CAD build for the part. Positions are in the model's coordinates, mm. Face numbers are marked on the shaded views. A direction names the side the tool comes from. Round coordinates to 2 decimals unless told otherwise and drop trailing zeros. Write each loop counter-clockwise with the first axis right and the second up, starting at its lowest first coordinate (ties: lowest second). Pieces come first, ordered by that corner, then holes. Notation, with made-up numbers: (51, 49) - (67, 49) arc R24 ccw to (67, 66) - close; hole circle Ø8 at (9, -36). An arc over 180 degrees is marked (long way). Use one line per item in the form item = value. Start each with the question number.
Item 1: Pull direction Z, two halves, no side cores. Call the marked faces 1, 2, 3 and 4: +Z half, -Z half, draft (parallel to the pull), parting line (faces both ways), or undercut.
Item 2: Band-saw the part on A-A, the plane x = -36. List the corners of the cut face in (y, z).
Item 3: Band-saw the part on D-D, the plane x = 1. List the corners of the cut face in (y, z).
Item 4: Band-saw the part on C-C, the plane z = -4.5. List the corners of the cut face in (x, y), and give its area (3 significant figures).
Item 5: Tool access for the marked faces 5, 6 and 7: list every direction of +Z, -Z, +X, -X, +Y, -Y with a clear straight run to the whole face (end or side of a thin tool).
Item 6: Drill centre lines: L1, parallel to X at y = 13, z = 30; L2, parallel to Z at x = -37, y = 12. Where is each one in solid material? Low to high.
Item 7: Pin check, flat tips, straight feed: pin 1 (4.5 mm diameter, centred on x = 37.5, z = -26.5, fed in from +Y); pin 2 (1.5 mm diameter, centred on y = 51, z = 21.5, fed in from +X); pin 3 (12 mm diameter, centred on x = -36.5, z = -33, fed in from +Y); pin 4 (3 mm diameter, centred on x = 27.5, z = -9.5, fed in from +Y). Stop position of each tip, or through.
Item 8: Band-saw the part on B-B, the plane y = 70. List the corners of the cut face in (x, z).
from build123d import *

# Parameters (mm, degrees)
BOSS_EXTRUDE1_DEPTH = 15
SKETCH1_5_R         = 7.5
CUT_EXTRUDE2_DEPTH  = 15
SKETCH1_6_R         = 7.5
SKETCH1_6_R_2       = 5.5
BOSS_EXTRUDE2_DEPTH = 10
BOSS_EXTRUDE3_DEPTH = 20


with BuildPart() as part:
    # Sketch1 → Boss-Extrude1 (new body)
    with BuildSketch(Plane(origin=(0, 0, 0), x_dir=(1, 0, 0), z_dir=(0, 1, 0))):
        with BuildLine():
            Line((52.75, -30), (52.75, 30))
            ThreePointArc((52.75, 30), (50.288021644, 38.233954897), (43.710264901, 43.765000629))
            Line((43.710264901, 43.765000629), (11.920529801, 57.530001258))
            ThreePointArc((11.920529801, 57.530001258), (0, 60), (-11.920529801, 57.530001258))
            Line((-11.920529801, 57.530001258), (-43.710264901, 43.765000629))
            ThreePointArc((-43.710264901, 43.765000629), (-50.288021644, 38.233954897), (-52.75, 30))
            Line((-52.75, 30), (-52.75, -30))
            ThreePointArc((-52.75, -30), (-48.356601718, -40.606601718), (-37.75, -45))
            Line((-37.75, -45), (37.75, -45))
            ThreePointArc((37.75, -45), (48.356601718, -40.606601718), (52.75, -30))
        make_face()
    extrude(amount=BOSS_EXTRUDE1_DEPTH)

    # Sketch1_5 → Cut-Extrude2 (cut)
    with BuildSketch(Plane(origin=(0, 0, 0), x_dir=(1, 0, 0), z_dir=(0, 1, 0))):
        with Locations((-37.75, 30)):
            Circle(SKETCH1_5_R)
        with Locations((37.75, 30)):
            Circle(SKETCH1_5_R)
        with Locations((37.75, -30)):
            Circle(SKETCH1_5_R)
        with Locations((-37.75, -30)):
            Circle(SKETCH1_5_R)
    extrude(amount=CUT_EXTRUDE2_DEPTH, mode=Mode.SUBTRACT)

    # Sketch1_6 → Boss-Extrude2 (add)
    with BuildSketch(Plane(origin=(0, 0, 0), x_dir=(1, 0, 0), z_dir=(0, 1, 0))):
        with Locations((-37.75, 30)):
            Circle(SKETCH1_6_R)
        with Locations((-37.75, 30)):
            Circle(SKETCH1_6_R_2, mode=Mode.SUBTRACT)
        with Locations((37.75, 30)):
            Circle(SKETCH1_6_R)
        with Locations((37.75, 30)):
            Circle(SKETCH1_6_R_2, mode=Mode.SUBTRACT)
        with Locations((37.75, -30)):
            Circle(SKETCH1_6_R)
        with Locations((37.75, -30)):
            Circle(SKETCH1_6_R_2, mode=Mode.SUBTRACT)
        with Locations((-37.75, -30)):
            Circle(SKETCH1_6_R)
        with Locations((-37.75, -30)):
            Circle(SKETCH1_6_R_2, mode=Mode.SUBTRACT)
    extrude(amount=BOSS_EXTRUDE2_DEPTH)

    # Sketch2 → Boss-Extrude3 (add, symmetric)
    with BuildSketch(Plane.XY):
        with BuildLine():
            Line((-25, 79), (-25, 76))
            ThreePointArc((-25, 76), (-25.292893219, 75.292893219), (-26, 75))
            Line((-26, 75), (-29.580398915, 75))
            ThreePointArc((-29.580398915, 75), (-26.457352845, 65.85756455), (-20.590457551, 58.181818182))
            ThreePointArc((-20.590457551, 58.181818182), (-14.516162744, 30.768138177), (-37.749172176, 15))
            Line((-37.749172176, 15), (37.749172176, 15))
            ThreePointArc((37.749172176, 15), (14.516162744, 30.768138177), (20.590457551, 58.181818182))
            ThreePointArc((20.590457551, 58.181818182), (26.457352845, 65.85756455), (29.580398915, 75))
            Line((29.580398915, 75), (26, 75))
            ThreePointArc((26, 75), (25.292893219, 75.292893219), (25, 76))
            Line((25, 76), (25, 79))
            ThreePointArc((25, 79), (24.707106781, 79.707106781), (24, 80))
            Line((24, 80), (22, 80))
            ThreePointArc((22, 80), (0, 58), (-22, 80))
            Line((-22, 80), (-24, 80))
            ThreePointArc((-24, 80), (-24.707106781, 79.707106781), (-25, 79))
        make_face()
    extrude(amount=BOSS_EXTRUDE3_DEPTH, both=True)


solid = part.part
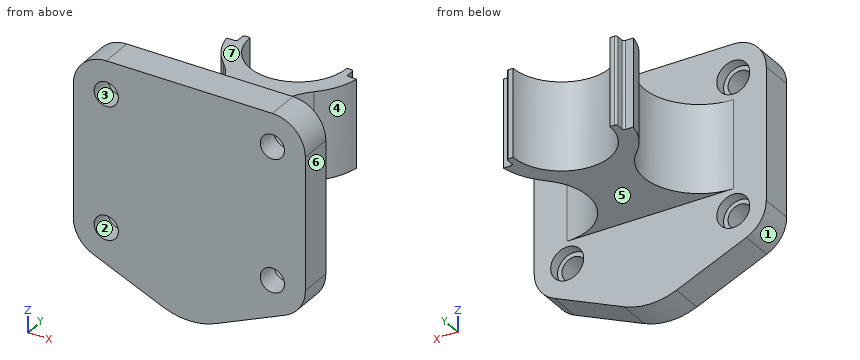
Determined:
q1.face_1 = -Z half
q1.face_2 = undercut
q1.face_3 = undercut
q1.face_4 = draft
q2.outline = (0, -47.1) - (15, -47.1) - (15, -37.29) - (10, -37.29) - (10, -35.21) - (0, -35.21) - close; (0, -24.79) - (10, -24.79) - (10, -22.71) - (15, -22.71) - (15, -20) - (15.06, -20) - (15.06, 20) - (15, 20) - (15, 22.71) - (10, 22.71) - (10, 24.79) - (0, 24.79) - close; (0, 35.21) - (10, 35.21) - (10, 37.29) - (15, 37.29) - (15, 45) - (0, 45) - close
q3.outline = (0, -59.98) - (15, -59.98) - (15, -20) - (58.02, -20) - (58.02, 20) - (15, 20) - (15, 45) - (0, 45) - close
q4.outline = (-52.75, 0) - (52.75, 0) - (52.75, 15) - (37.75, 15) arc R25 cw to (20.59, 58.18) arc R30 ccw to (29.58, 75) - (26, 75) arc R1 cw to (25, 76) - (25, 79) arc R1 ccw to (24, 80) - (22, 80) arc R22 cw to (-22, 80) - (-24, 80) arc R1 ccw to (-25, 79) - (-25, 76) arc R1 cw to (-26, 75) - (-29.58, 75) arc R30 ccw to (-20.59, 58.18) arc R25 cw to (-37.75, 15) - (-52.75, 15) - close
q4.area = 3,410 mm²
q5.face_5 = -Z, +X, -X, +Y
q5.face_6 = +Z, -Z, +X, +Y, -Y
q5.face_7 = +Z, +X, -X, +Y
q6.L1 = -52.75 to -45.25, -30.25 to 30.25, 45.25 to 52.75
q6.L2 = -46.67 to -37.46, -22.54 to 22.54, 37.46 to 45
q7.pin_1 = 10
q7.pin_2 = through
q7.pin_3 = 15
q7.pin_4 = 75
q8.outline = (-28.28, -20) - (-19.6, -20) - (-19.6, 20) - (-28.28, 20) - close; (19.6, -20) - (28.28, -20) - (28.28, 20) - (19.6, 20) - close
